Model file for the job. Use its own axes, mm. A direction names the side the tool comes from. Give positions to 0.01 mm unless a question says otherwise; leave off trailing zeros. Write each loop counter-clockwise with the first axis right and the second up, starting at its lowest first coordinate (ties: lowest second). Pieces come first, ordered by that corner, then holes. Notation, with made-up numbers: M 4.25,60.5 L 15.25,60.5 A21 ccw 15.25,64.5 Z; hole C 33.25,89 d4. An arc over 180 degrees is marked long. Answer as a JSON object with one key per item and string values. Group by question number.
Autodesk Inventor part; units mm, degrees
ref_plane "YZ Plane" through (0, 0, 0) normal (1, 0, 0) x (0, 1, 0)
ref_plane "XZ Plane" through (0, 0, 0) normal (0, 1, 0) x (-1, 0, 0)
ref_plane "XY Plane" through (0, 0, 0) normal (0, 0, 1) x (1, 0, 0)
sketch "스케치1" plane through (0, 0, 0) normal (0, 1, 0) x (-1, 0, 0)
  line L0 (60, 80) -> (-60, 80)
  line L1 (-60, 80) -> (-60, -80)
  line L2 (-60, -80) -> (60, -80)
  line L3 (60, -80) -> (60, 80)
  line L4 (60, 80) -> (-60, -80) construction
  line L5 (-60, 80) -> (60, -80) construction
  point P0 (0, 0)
  dimension "d0" = 120
  dimension "d1" = 160
extrude "돌출1" add sketch "스케치1" along normal blind 60
sketch "스케치2" plane through (0, 60, 0) normal (0, 1, 0) x (1, 0, 0)
  line L0 (60, -80) -> (60, 80)
  line L1 (60, 80) -> (-60, 80)
  line L2 (55, 102.1646) -> (-55, 102.1646)
  line L3 (-55, 102.1646) -> (-55, -89.711)
  line L4 (-55, -89.711) -> (55, -89.711)
  line L5 (55, -89.711) -> (55, 102.1646)
  line L6 (-60, 80) -> (-60, -80)
  point P0 (0, 0)
  point P1 (55, 80)
  point P2 (-55, 80)
  dimension "d6" = 5
  dimension "d7" = 5
extrude "돌출2" cut sketch "스케치2" against normal blind 40 contours L5 L4 L3 L1
sketch "스케치12" plane through (60, 0, -80) normal (0, 0, -1) x (-1, 0, 0)
  line L0 (-34.8463, 10) -> (156.2634, 10)
  line L1 (156.2634, 10) -> (156.2634, -36.9465)
  line L2 (156.2634, -36.9465) -> (-34.8463, -36.9465)
  line L3 (-34.8463, -36.9465) -> (-34.8463, 10)
  line L4 (0, 0) -> (120, 0)
  point P0 (60, 0)
  dimension "d85" = 10
extrude "돌출10" cut sketch "스케치12" against normal through all
sketch "스케치13" plane through (-55, 20, 80) normal (0, 0, 1) x (1, 0, 0)
  line L0 (0, 40) -> (0, 0)
  line L1 (0, 0) -> (110, 0)
  line L2 (0, 40) -> (110, 40)
  line L3 (110, 40) -> (110, 0)
  line L4 (110, 0) -> (0, 0)
  line L5 (0, 0) -> (0, 40)
  point P0 (55, -20)
extrude "돌출11" add sketch "스케치13" against normal blind 5
sketch "스케치14" plane through (55, 20, -80) normal (0, 0, -1) x (-1, 0, 0)
  line L0 (0, 0) -> (0, 40)
  line L1 (110, 0) -> (0, 0)
  line L2 (0, 40) -> (110, 40)
  line L3 (110, 40) -> (110, 0)
  line L4 (110, 0) -> (0, 0)
  line L5 (0, 0) -> (0, 40)
  point P0 (55, -20)
extrude "돌출12" add sketch "스케치14" against normal blind 5
sketch "스케치15" plane through (60, 60, -80) normal (0, 0, -1) x (-1, 0, 0)
  point P0 (60, -60)
sketch "스케치16" plane through (60, 60, -80) normal (0, 0, -1) x (-1, 0, 0)
  point P0 (60, -60)
sketch "스케치17" plane through (0, 20, 0) normal (0, 1, 0) x (1, 0, 0)
  line L0 (7, 27) -> (45, 27)
  line L1 (45, 27) -> (45, 65)
  line L2 (45, 65) -> (7, 65)
  line L3 (7, 65) -> (7, 27)
  line L4 (55, 75) -> (55, -75)
  line L5 (55, 75) -> (-55, 75)
  circle A0 centre (7, 27) radius 1.6
  circle A1 centre (7, 65) radius 1.6
  circle A2 centre (45, 65) radius 1.6
  circle A3 centre (45, 27) radius 1.6
  line L6 (-47.9371, 14.7215) -> (-7.9371, 14.7215)
  line L7 (-7.9371, 14.7215) -> (-7.9371, 64.7215)
  line L8 (-7.9371, 64.7215) -> (-47.9371, 64.7215)
  line L9 (-47.9371, 64.7215) -> (-47.9371, 14.7215)
  point P0 (0, 0)
  dimension "d92" = 38
  dimension "d93" = 38
  dimension "d95" = 10
  dimension "d96" = 10
  dimension "d97" = 3.2
  dimension "d98" = 3.2
  dimension "d99" = 3.2
  dimension "d100" = 3.2
  dimension "d113" = 40
  dimension "d114" = 50
extrude "돌출13" cut sketch "스케치17" against normal through all contours L3 A0 L0 | L0 A0 L3 | A3 L1 L0 | L0 L1 A3 | A1 L2 L3 | L3 L2 A1 | A2 L2 L1 | L1 L2 A2
sketch "스케치19" plane through (60, 60, -80) normal (0, 0, -1) x (-1, 0, 0)
  line L0 (5, -40) -> (115, -40)
  circle A0 centre (46.5, -35) radius 8.5
  circle A1 centre (73.5, -35) radius 8.5
  line L1 (5, 0) -> (5, -40)
  line L2 (115, -40) -> (115, 0)
  point P0 (60, -60)
  dimension "d105" = 27
  dimension "d106" = 41.5
  dimension "d107" = 17
  dimension "d108" = 17
  dimension "d109" = 5
  dimension "d110" = 5
extrude "돌출14" cut sketch "스케치19" against normal through all
sketch "스케치21" plane through (0, 20, 0) normal (0, 1, 0) x (1, 0, 0)
  circle A0 centre (5.4243, 8.1678) radius 7.5
  line L0 (-49.3888, 17.2731) -> (-9.3888, 17.2731)
  line L1 (-9.3888, 17.2731) -> (-9.3888, 67.2731)
  line L2 (-9.3888, 67.2731) -> (-49.3888, 67.2731)
  line L3 (-49.3888, 67.2731) -> (-49.3888, 17.2731)
  point P0 (0, 0)
  dimension "d117" = 15
  dimension "d118" = 50
  dimension "d119" = 40
extrude "돌출15" cut sketch "스케치21" against normal through all contours A0
sketch "스케치23" plane through (0, 20, 0) normal (0, 1, 0) x (1, 0, 0)
  line L0 (-48.6, -65) -> (20, -65)
  line L1 (20, -65) -> (20, -11.6)
  line L2 (20, -11.6) -> (-48.6, -11.6)
  line L3 (-48.6, -11.6) -> (-48.6, -65)
  line L4 (55, 75) -> (55, -75)
  line L5 (-55, -75) -> (55, -75)
  circle A0 centre (4.7, -62.45) radius 1.6
  circle A1 centre (6.03, -14.15) radius 1.6
  circle A2 centre (-46.05, -47.16) radius 1.6
  circle A3 centre (-46.05, -19.23) radius 1.6
  point P0 (0, 0)
  dimension "d123" = 68.6
  dimension "d124" = 53.4
  dimension "d125" = 35
  dimension "d126" = 10
  dimension "d127" = 3.2
  dimension "d128" = 15.3
  dimension "d129" = 2.55
  dimension "d130" = 3.2
  dimension "d131" = 13.97
  dimension "d132" = 2.55
  dimension "d133" = 3.2
  dimension "d134" = 35.56
  dimension "d135" = 3.2
  dimension "d136" = 2.55
  dimension "d137" = 2.55
  dimension "d138" = 7.63
extrude "돌출16" cut sketch "스케치23" against normal through all contours A0 | A1 | A2 | A3
sketch "스케치24" plane through (0, 20, 0) normal (0, 1, 0) x (1, 0, 0)
  line L0 (-55, -75) -> (55, -75)
  line L1 (55, 75) -> (55, -75)
  line L2 (-55, -75) -> (55, -75)
  line L3 (55, -75) -> (55, 75)
  line L4 (55, 75) -> (-55, 75)
  line L5 (-55, 75) -> (-55, -75)
  point P0 (0, 0)
extrude "돌출17" cut sketch "스케치24" against normal through all
sketch "스케치25" plane through (0, 60, 0) normal (0, 1, 0) x (1, 0, 0)
  line L0 (-60, 80) -> (-60, -80)
  line L1 (60, -80) -> (60, 80)
  line L2 (-60, 80) -> (60, 80)
  line L3 (60, 80) -> (60, -77)
  line L4 (60, -77) -> (-60, -77)
  line L5 (-60, -77) -> (-60, 80)
  line L6 (-60, -80) -> (60, -80)
  point P0 (0, 0)
  dimension "d143" = 3
extrude "돌출18" cut sketch "스케치25" against normal through all contours L2 L1 L4 L0
sketch "스케치26" plane through (-60, 60, 80) normal (0, 0, 1) x (1, 0, 0)
  line L0 (120, -50) -> (120, 0)
  line L1 (0, -50) -> (120, -50)
  line L2 (45, -50) -> (75, -50)
  line L3 (75, -50) -> (75, -53)
  line L4 (75, -53) -> (45, -53)
  line L5 (45, -53) -> (45, -50)
  dimension "d149" = 3
extrude "돌출19" add sketch "스케치26" against normal blind 3
sketch "스케치27" plane through (-60, 60, 80) normal (0, 0, 1) x (1, 0, 0)
  line L0 (116.8483, -15) -> (123, -15)
  line L1 (123, -15) -> (123, -35)
  line L2 (123, -35) -> (116.8483, -35)
  line L3 (116.8483, -35) -> (116.8483, -15)
  line L4 (0, 0) -> (120, 0)
  line L5 (120, -50) -> (120, 0)
  point P0 (60, -60)
  point P1 (120, -15)
  point P2 (120, -35)
  dimension "d152" = 20
  dimension "d153" = 15
  dimension "d154" = 3
extrude "돌출20" add sketch "스케치27" against normal blind 3 contours L0 L1 L2 L5
mirror "미러3" about plane through (0, 0, 0) normal (1, 0, 0) of "돌출20"
sketch "스케치28" plane through (-60, 60, 80) normal (0, 0, 1) x (1, 0, 0)
  line L0 (44.5, 7.1302) -> (75.5, 7.1302)
  line L1 (75.5, 7.1302) -> (75.5, -3)
  line L2 (75.5, -3) -> (44.5, -3)
  line L3 (44.5, -3) -> (44.5, 7.1302)
  line L4 (120, -15) -> (120, 0)
  line L5 (0, 0) -> (120, 0)
  point P0 (60, -60)
  point P1 (75.5, 0)
  point P2 (44.5, 0)
  dimension "d157" = 31
  dimension "d158" = 44.5
  dimension "d159" = 3
extrude "돌출21" cut sketch "스케치28" against normal through all contours L5 L1 L2 L3
sketch "스케치29" plane through (60, 10, 77) normal (0, 0, -1) x (-1, 0, 0)
  line L0 (117, 54.1407) -> (145.6874, 54.1407)
  line L1 (145.6874, 54.1407) -> (145.6874, -6.9321)
  line L2 (145.6874, -6.9321) -> (117, -6.9321)
  line L3 (117, -6.9321) -> (117, 54.1407)
  line L4 (120, 50) -> (120, 35)
  line L5 (44.5, 47) -> (75.5, 47)
  line L6 (60, 47) -> (60, -3)
  line L7 (45, -3) -> (75, -3)
  line L8 (3, 54.1407) -> (-25.6874, 54.1407)
  line L9 (-25.6874, 54.1407) -> (-25.6874, -6.9321)
  line L10 (-25.6874, -6.9321) -> (3, -6.9321)
  line L11 (3, -6.9321) -> (3, 54.1407)
  line L12 (0, 50) -> (0, 35)
  point P0 (60, -10)
  dimension "d162" = 3
extrude "돌출22" cut sketch "스케치29" against normal through all
sketch "스케치30" plane through (15, 7, 77) normal (0, 0, -1) x (-1, 0, 0)
  line L0 (64.5699, 38) -> (75, 38)
  line L1 (75, 38) -> (75, 18)
  line L2 (75, 18) -> (64.5699, 18)
  line L3 (64.5699, 18) -> (64.5699, 38)
  line L4 (30.5, 53) -> (72, 53)
  line L5 (72, 3) -> (72, 53)
  line L6 (-0.5, 50) -> (30.5, 50)
  line L7 (15, 50) -> (15, 0)
  line L8 (30, 0) -> (0, 0)
  line L9 (-34.5699, 38) -> (-45, 38)
  line L10 (-45, 38) -> (-45, 18)
  line L11 (-45, 18) -> (-34.5699, 18)
  line L12 (-34.5699, 18) -> (-34.5699, 38)
  line L13 (-42, 53) -> (-42, 3)
  point P0 (15, -7)
  point P1 (72, 38)
  point P2 (72, 18)
  point P3 (-42, 18)
  point P4 (-42, 38)
  dimension "d165" = 20
  dimension "d166" = 15
  dimension "d167" = 3
extrude "돌출23" add sketch "스케치30" against normal blind 3 contours L0 L1 L2 L5 | L13 L11 L10 L9
sketch "스케치31" plane through (-15, 7, 80) normal (0, 0, 1) x (1, 0, 0)
  point P0 (15, -7)
properties part number "본체 겉면 레이저 앞판"
Q1. Two-plate mould, pull along X, no slides. Class faces 6 (the flat face through (15.5, 59, 79)), 7 (the flat face through (60, 35, 78)), 8 (the flat face through (59, 25, 78)): +X half, -X half, draft (parallel to the pull), parting line (faces both ways), or undercut.
Q2. Slice it at B-B, the plane z = 78.1. Write the cut outline in (x, y).
Q3. Drop flat-ended pins along their axis: P1, Ø1.5, axis at y = 8, z = 78.5, coming from the +X side; P2, Ø22, axis at x = 13.5, y = 25, coming from the +Z side; P3, Ø1.5, axis at x = 6.5, z = 78.5, coming from the +Y side; P4, Ø0.9, axis at y = 9, z = 78, coming from the -X side. Give the stop position or say it passes through.
Q4. Slice it at D-D, the plane y = 52. Write the cut outline in (x, z).
Q5. 3-axis set-ups, long thin cutter, end or side, ignore diameter. For faces 1 (the flat face through (-59, 25, 78)), 2 (the flat face through (0, 7, 79)), 3 (the flat face through (-57, 52, 78)), 4 (the flat face through (0, 57, 79)), 5 (the flat face through (58, 45, 78)): which of +Z, -Z, +X, -X, +Y, -Y reach the whole face in a straight line?
Q6. Slice it at A-A, the plane x = 13.5. Write the cut outline in (y, z).
Q7. Wall check: L1, parallel to Y at x = 14, z = 77.65; L2, parallel to X at y = 28.5, z = 79.75; L3, parallel to X at y = 21.5, z = 78. Give the ranges that are in metal, low to high.
Q8. Slice it at C-C, the plane x = -3.5. Write the cut outline in (y, z).
Solved:
{
 "1": {"face 6": "undercut", "face 7": "+X half", "face 8": "draft"},
 "2": {"outline": "M -60,25 L -57,25 L -57,10 L -15,10 L -15,7 L 15,7 L 15,10 L 57,10 L 57,25 L 60,25 L 60,45 L 57,45 L 57,60 L 15.5,60 L 15.5,57 L -15.5,57 L -15.5,60 L -57,60 L -57,45 L -60,45 Z; hole C -13.5,25 d17; hole C 13.5,25 d17"},
 "3": {"P1": "stops at x = 15", "P2": "stops at z = 80", "P3": "stops at y = 57", "P4": "stops at x = -15"},
 "4": {"outline": "M -57,77 L 57,77 L 57,80 L -57,80 Z"},
 "5": {"face 1": "+Z, -Z, -X, -Y", "face 2": "+Z, -Z, +X, -X, -Y", "face 3": "+Z, -Z, -X, +Y", "face 4": "+Z, -Z, +Y", "face 5": "+Z, -Z, +X, +Y"},
 "6": {"outline": "M 7,77 L 16.5,77 L 16.5,80 L 7,80 Z; M 33.5,77 L 57,77 L 57,80 L 33.5,80 Z"},
 "7": {"L1": "y = 7 to 16.51, 33.49 to 57", "L2": "x = -60 to -21.25, -5.75 to 5.75, 21.25 to 60", "L3": "x = -57 to -21.25, -5.75 to 5.75, 21.25 to 57"},
 "8": {"outline": "M 7,77 L 57,77 L 57,80 L 7,80 Z"}
}
